```python
from build123d import *

# Parameters (mm, degrees)
SKETCH1_R           = 2.5
SKETCH1_R_2         = 1
BOSS_EXTRUDE1_DEPTH = 3


with BuildPart() as part:
    # Sketch1 → Boss-Extrude1 (new body)
    with BuildSketch(Plane(origin=(0, 0, 0), x_dir=(0, 0, -1), z_dir=(1, 0, 0))):
        with BuildLine():
            Line((-81.371714004, 9.04040404), (7.575757576, 9.04040404))
            ThreePointArc((7.575757576, 9.04040404), (14.646825388, 6.111471852), (17.575757576, -0.95959596))
            ThreePointArc((17.575757576, -0.95959596), (14.646825388, -8.030663771), (7.575757576, -10.95959596))
            Line((7.575757576, -10.95959596), (-81.897978214, -10.95959596))
            ThreePointArc((-81.897978214, -10.95959596), (-89.232178131, -8.139656658), (-92.424242424, -0.95959596))
            ThreePointArc((-92.424242424, -0.95959596), (-88.969046026, 6.329457626), (-81.371714004, 9.04040404))
        make_face()
        with Locations((7.575757576, -0.95959596)):
            Circle(SKETCH1_R, mode=Mode.SUBTRACT)
        with Locations((12.575757576, -0.95959596)):
            Circle(SKETCH1_R_2, mode=Mode.SUBTRACT)
        with Locations((2.575757576, -0.95959596)):
            Circle(SKETCH1_R_2, mode=Mode.SUBTRACT)
    extrude(amount=BOSS_EXTRUDE1_DEPTH)


solid = part.part
```
Read the model definition and answer for the solid it produces. Units are mm, in the model's axes. Round coordinates to 2 decimals unless told otherwise and drop trailing zeros. Write each loop counter-clockwise with the first axis right and the second up, starting at its lowest first coordinate (ties: lowest second). Pieces come first, ordered by that corner, then holes. Notation, with made-up numbers: (-24.5, 68.5) -> (5.5, 68.5) arc R23 ccw to (5.5, 100.5) -> close; hole circle Ø9 at (79.25, -25). An arc over 180 degrees is marked (long way). Answer in a Markdown table with one row per item. Add a question column.
1) Find section B-B, the plane y = -6.5. Determine the outline of the cut face in (x, z).
2) Determine the mould class of faces 1 (the face through (1.479, -8.217, 89.15)), 2 (the face through (1.479, -1.917, -9.885)), 3 (the face through (0, -1, 37)), 4 (the face through (1.479, -0.916, -11.577)) for opening direction Y: pulls with the +Y half, pulls with the -Y half, needs draft (parallel to the pull), parting line crosses it, or undercut.
3) Find section A-A, the plane x = 1.75. Determine the outline of the cut face in (y, z), and give its area (3 significant figures).
4) Find section C-C, the plane y = 5.25. Determine the outline of the cut face in (x, z), and give its area (3 significant figures).
5) Consider line 1 (Z direction, x = 0.3, y = -1.5); line 2 (Z direction, x = 1.7, y = -1.75); line 3 (Y direction, x = 1.35, z = 34). Determine where each line is inside the solid, lowest interval first.
6) Given P1, Ø1.5, axis at x = 2, z = 34, coming from the +Y side; P2, Ø1, axis at x = 1.5, y = -4, coming from the +Z side; P3, Ø1.5, axis at x = 2, z = 35, coming from the -Y side; P4, Ø1.2, axis at y = -0.96, z = -12.58, coming from the +X side (1 decimal), each flat-ended and moving along its own axis, determine where each tip first touches the part or whether it passes through.
Findings below:
| question | item | result |
|---|---|---|
| 1 | outline | (0, -15.9) -> (3, -15.9) -> (3, 90.63) -> (0, 90.63) -> close |
| 2 | face 1 | pulls with the -Y half |
| 2 | face 2 | undercut |
| 2 | face 3 | needs draft |
| 2 | face 4 | undercut |
| 3 | outline | (-10.96, -7.58) arc R10 ccw to (9.04, -7.58) -> (9.04, 81.37) arc R10.54 ccw to (-0.96, 92.42) arc R10.27 ccw to (-10.96, 81.9) -> close; hole circle Ø5 at (-0.96, -7.58); hole circle Ø2 at (-0.96, -12.58); hole circle Ø2 at (-0.96, -2.58) |
| 3 | area | 2,090 mm² |
| 4 | outline | (0, -15.41) -> (3, -15.41) -> (3, 90) -> (0, 90) -> close |
| 4 | area | 316 mm² |
| 5 | line 1 | -17.56 to -13.42, -11.73 to -10.02, -5.13 to -3.42, -1.73 to 92.4 |
| 5 | line 2 | -17.54 to -13.19, -11.96 to -9.95, -5.2 to -3.19, -1.96 to 92.37 |
| 5 | line 3 | -10.96 to 9.04 |
| 6 | P1 | y = 9.04 |
| 6 | P2 | z = 92.04 |
| 6 | P3 | y = -10.96 |
| 6 | P4 | through |
